The listing builds one solid part. Answer for the finished solid, in the listing's coordinates (mm). Face numbers are marked on the shaded views. A direction names the side the tool comes from. Round coordinates to 2 decimals unless told otherwise and drop trailing zeros. Loops run counter-clockwise (first coordinate to the right, second up) from the corner with the lowest first, then second, coordinate; pieces in that order, holes last. Notation, with made-up numbers: M -29,-2 L -11,-2 A10 ccw -11,6 Z; hole C -28,5.25 d11. An arc over 180 degrees is marked long. Put each result on its own line as item: value. Start each with the question number.
(1) Straight lines are drawn through the part: line 1 (Y direction, x = -1.5, z = -6.25); line 2 (Z direction, x = 35.5, y = 4); line 3 (X direction, y = 15.75, z = 7.5). For each, find the intervals that lie inside material, in ascending order.
(2) Section A-A, the plane y = 4 is taken. Determine the outline of the cut face in (x, z).
(3) Determine the mould class of the marked faces 3, 4 and 5 for opening direction Y: released by +Y, released by -Y, zero draft, split by the parting line, or undercut.
(4) Section D-D, the plane x = -3 is taken. Determine the outline of the cut face in (y, z), then the cut area to 3 significant figures.
(5) Section B-B, the plane z = 1.75 is taken. Determine the outline of the cut face in (x, y), then the cut area to 3 significant figures.
(6) Flat-ended cylindrical pins translate along their axes: P1, Ø8, axis at y = 5.5, z = -1.5, coming from the +X side; P2, Ø6, axis at y = 20.5, z = 5, coming from the +X side; P3, Ø2, axis at y = 17, z = -11.5, coming from the +X side; P4, Ø6, axis at x = -9, y = 2.5, coming from the +Z side. Find the tip coordinate at first contact, or state that the pin passes through.
(7) Section C-C, the plane y = 10 is taken. Determine the outline of the cut face in (x, z).
(8) Which of the six approach directions +Z, -Z, +X, -X, +Y, -Y give full straight-line access (tool end or side, diameter ignored) to the marked faces 1 and 2?
```python
from build123d import *

# Parameters (mm, degrees)
BOSS_EXTRUDE1_DEPTH = 25
SHELL1_T            = -2
SKETCH2_R           = 6.35
CUT_EXTRUDE1_DEPTH  = 10


with BuildPart() as part:
    # Sketch1 → Boss-Extrude1 (new body)
    with BuildSketch(Plane(origin=(0, 0, 0), x_dir=(1, 0, 0), z_dir=(0, 1, 0))):
        Polygon((-17.350316623, 15.957783641), (45.649683377, 15.957783641), (20.279683377, -9.042216359), (8.019683377, -9.042216359), align=None)
    extrude(amount=BOSS_EXTRUDE1_DEPTH)

    # Shell1
    shell1_openings = [part.faces().sort_by_distance(p)[0] for p in [
        (32.964683377, 12.5, -3.457783641),
        (-4.665316623, 12.5, -3.457783641),
    ]]
    offset(amount=SHELL1_T, openings=shell1_openings, kind=Kind.INTERSECTION)

    # Sketch2 → Cut-Extrude1 (cut)
    with BuildSketch(Plane(origin=(0, 0, -15.957783641), x_dir=(-1, 0, 0), z_dir=(0, 0, -1))):
        with Locations((-14.149683377, 12.5)):
            Circle(SKETCH2_R)
    extrude(amount=-CUT_EXTRUDE1_DEPTH, mode=Mode.SUBTRACT)


solid = part.part
```
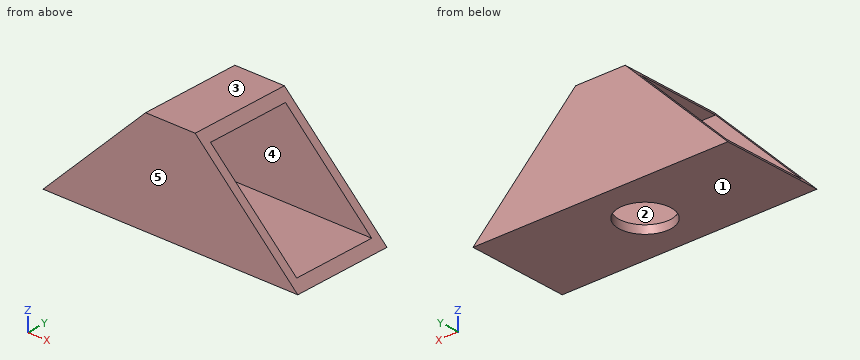
Recorded:
1. line 1: y = 0 to 2, 23 to 25
1. line 2: z = -15.96 to -13.96
1. line 3: x = 6.45 to 21.84
2. outline: M -17.35,-15.96 L 45.65,-15.96 L 43.62,-13.96 L -15.32,-13.96 Z; M 5.99,7.04 L 22.31,7.04 L 20.28,9.04 L 8.02,9.04 Z
3. face 3: zero draft
3. face 4: undercut
3. face 5: released by -Y
4. outline: M 0,-15.96 L 25,-15.96 L 25,-1.82 L 23,-1.82 L 23,-13.96 L 2,-13.96 L 2,-1.82 L 0,-1.82 Z
4. area: 98.6 mm²
5. outline: M 0.62,0 L 27.68,0 L 27.68,2 L 0.62,2 Z; M 0.62,23 L 27.68,23 L 27.68,25 L 0.62,25 Z
5. area: 108 mm²
6. P1: stops at x = 32.94
6. P2: stops at x = 26.06
6. P3: passes through
6. P4: stops at z = -4.81
7. outline: M -17.35,-15.96 L 8.31,-15.96 L 8.31,-13.96 L -15.32,-13.96 Z; M 5.99,7.04 L 22.31,7.04 L 20.28,9.04 L 8.02,9.04 Z; M 19.99,-15.96 L 45.65,-15.96 L 43.62,-13.96 L 19.99,-13.96 Z
8. face 1: -Z, +X, -X, +Y, -Y
8. face 2: +X, -X
